Answer from the drawing. Dimensions are ordinates in mm from the lowest x, y and z of the part. A direction names the side the tool comes from. Give positions to 0.01 mm unless a question says otherwise; leave off trailing zeros. Loops run counter-clockwise (first coordinate to the right, second up) from the corner with the lowest first, then second, coordinate; pieces in that order, holes last. Notation, with made-up numbers: (29.5, 5.25) - (66.5, 5.25) arc R18 ccw to (66.5, 25.25) - close; hole circle Ø7 at (-3.75, -8). An arc over 180 degrees is marked (long way). Answer as CSV lines item,"result". Start each with the question number.
1) A cutting plane is placed at B-B (z = 10). Determine the outline of the cut face in (x, y).
2) Flat-ended cylindrical pins translate along their axes: pin 1 (5 mm diameter, centred on x = 1.5, y = 6, fed in from +Z); pin 2 (3.5 mm diameter, centred on x = 29.5, y = 7.5, fed in from -Z); pin 3 (3 mm diameter, centred on y = 8, z = 22, fed in from -X). Find the tip coordinate at first contact, or state that the pin passes through.
3) For the marked faces 1, 2, 3, 4 and 5, determine the directions among +Z, -Z, +X, -X, +Y, -Y from which every point of the face is accessible in a straight line to the end or side of a thin tool.
4) A cutting plane is placed at A-A (x = 16.5). Determine the outline of the cut face in (y, z).
5) Find the intervals of material crossed by line 1 along X through (y, z) = (1.5, 19.5); line 2 along Z through (x, y) = (28, 7); line 3 along Z through (x, y) = (16, 4.25), in increasing order.
6) A cutting plane is placed at C-C (y = 2). Determine the outline of the cut face in (x, z).
7) A cutting plane is placed at D-D (x = 2). Determine the outline of the cut face in (y, z).
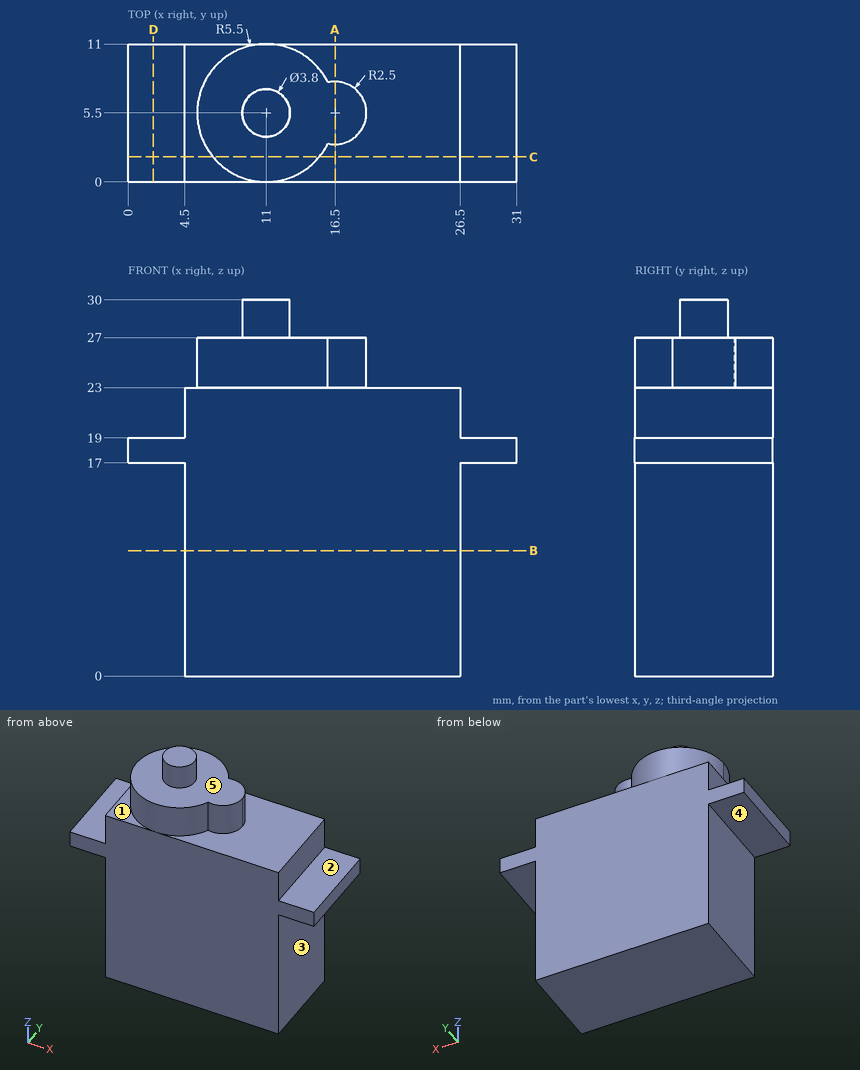
Ans:
1,outline,"(4.5, 0) - (26.5, 0) - (26.5, 11) - (4.5, 11) - close"
2,pin 1,"z = 19"
2,pin 2,"z = 17"
2,pin 3,"x = 4.5"
3,face 1,"+Z, -X"
3,face 2,"+Z, +X, +Y, -Y"
3,face 3,"-Z, +X, +Y, -Y"
3,face 4,"-Z, -X, +Y, -Y"
3,face 5,"+Z"
4,outline,"(0, 0) - (11, 0) - (11, 23) - (8, 23) - (8, 27) - (3, 27) - (3, 23) - (0, 23) - close"
5,line 1,"4.5 to 26.5"
5,line 2,"17 to 19"
5,line 3,"0 to 27"
6,outline,"(0, 17) - (4.5, 17) - (4.5, 0) - (26.5, 0) - (26.5, 17) - (31, 17) - (31, 19) - (26.5, 19) - (26.5, 23) - (15.24, 23) - (15.24, 27) - (6.76, 27) - (6.76, 23) - (4.5, 23) - (4.5, 19) - (0, 19) - close"
7,outline,"(0, 17) - (11, 17) - (11, 19) - (0, 19) - close"
